Here's how the part is built. I have some questions about the finished solid (model axes, mm). A direction names the side the tool comes from. Round coordinates to 2 decimals unless told otherwise and drop trailing zeros. Write each loop counter-clockwise with the first axis right and the second up, starting at its lowest first coordinate (ties: lowest second). Pieces come first, ordered by that corner, then holes. Notation, with made-up numbers: (72, 59.5) - (108, 59.5) arc R4 ccw to (108, 65.5) - close; hole circle Ø2 at (43.5, 28.25). An arc over 180 degrees is marked (long way). One line per item, written item: value. Start each with the question number.
Item 1: For P1, Ø10, axis at x = 81, y = -48.5, coming from the +Z side; P2, Ø1.5, axis at y = -12.5, z = 15.5, coming from the +X side; P3, Ø1.5, axis at y = 14, z = 30, coming from the +X side; P4, Ø12, axis at y = -67.5, z = 10.5, coming from the +X side, each with a flat end and sliding along its axis, tell me the tip position at first contact or that it passes through.
Item 2: Imagine slicing it at B-B, the plane z = -13.5. Please give me the cut outline in (x, y).
Item 3: If I drill on line 1 (Z direction, x = -35, y = -20.5); line 2 (X direction, y = -64, z = 1); line 3 (Z direction, x = -42.5, y = -14.5), over which ranges is the centre line in solid material (lowest first)?
Item 4: Imagine slicing it at C-C, the plane x = 33.5. Please give me the cut outline in (y, z), then the cut area to 3 significant figures.
Item 5: Imagine slicing it at A-A, the plane y = 27. Please give me the cut outline in (x, z), then the cut area to 3 significant figures.
Item 6: Imagine slicing it at D-D, the plane x = -58. Please give me the cut outline in (y, z), then the cut area to 3 significant figures.
Item 7: Thinking about a two-plate mould opening in X: for faces 5 (the face through (59.417, -33.844, -12.525)), 6 (the face through (-30, 0, 28.945)), 7 (the face through (21.498, -69, 1)), which applies, released by +X, released by -X, zero draft, split by the parting line, or undercut?
Item 8: For faces 1 (the face through (-30, 16.289, 33)), 2 (the face through (53, -61.088, -4)), 3 (the face through (23.58, -33.81, -4.68)), 4 (the face through (0, -1, -16)), which set-ups out of +Z, -Z, +X, -X, +Y, -Y let a thin tool reach every point of the face, with its end or its side?
```python
from build123d import *

# Parameters (mm, degrees)
F1_DEPTH  = 76.2
F2_DEPTH  = 76.2
F3_W      = 72.8542578737
F3_H      = 12.1001238003
F4_DEPTH  = 152.401
F5_W      = 82.1163672954
F5_H      = 15.1120005071
F6_DEPTH  = 59.4443229417
F7_W      = 32.5772352517
F7_H      = 8.1773027778
F8_DEPTH  = 176.4699010899
F9_R      = 11.4001375148
F10_DEPTH = 59.4443229417
F11_R     = 12.1676085245
F12_DEPTH = 59.4443229417
F13_R     = 11.1566059008
F14_DEPTH = 59.4443229417
F15_R     = 11.1566059008
F16_DEPTH = 59.4443229417


with BuildPart() as f1:
    # F0 (on Front) → F1 (new body)
    with BuildSketch(Plane.XZ):
        Polygon((103.6146432161, -22.3206151277), (0, 37.122707814), (-72.8542578737, 37.122707814), (-72.8542578737, -22.3206151277), align=None)
    extrude(amount=F1_DEPTH)

    # F2 (add): a face of the model
    f2_faces = [f1.faces().sort_by_distance(p)[0] for p in [
        (-6.935088319, 0, 3.283766903),
    ]]
    extrude(f2_faces, amount=F2_DEPTH)

    # F3 (on face) → F4 (cut, through all)
    with BuildSketch(Plane.XZ.offset(76.2)):
        with Locations((-36.4271289369, -16.2705532275)):
            Rectangle(F3_W, F3_H)
    extrude(amount=-F4_DEPTH, mode=Mode.SUBTRACT)

    # F5 (on face) → F6 (cut, through all)
    with BuildSketch(Plane(origin=(0, 0, -22.3206151277), x_dir=(1, 0, 0), z_dir=(0, 0, -1))):
        with Locations((62.5564595684, 68.6439997464)):
            Rectangle(F5_W, F5_H)
    extrude(amount=-F6_DEPTH, mode=Mode.SUBTRACT)

    # F7 (on face) → F8 (cut, through all)
    with BuildSketch(Plane(origin=(-72.8542578737, 0, 0), x_dir=(0, -1, 0), z_dir=(-1, 0, 0))):
        with Locations((0, 33.0340564251)):
            Rectangle(F7_W, F7_H)
    extrude(amount=-F8_DEPTH, mode=Mode.SUBTRACT)

    # F9 (on face) → F10 (cut, through all)
    with BuildSketch(Plane(origin=(0, 0, -22.3206151277), x_dir=(1, 0, 0), z_dir=(0, 0, -1))):
        with Locations((34.9696464837, 33.3093106747)):
            Circle(F9_R)
    extrude(amount=-F10_DEPTH, mode=Mode.SUBTRACT)

    # F11 (on face) → F12 (cut, through all)
    with BuildSketch(Plane(origin=(0, 0, -22.3206151277), x_dir=(1, 0, 0), z_dir=(0, 0, -1))):
        with Locations((71.5732872486, 33.3093106747)):
            Circle(F11_R)
    extrude(amount=-F12_DEPTH, mode=Mode.SUBTRACT)

    # F13 (on face) → F14 (cut, through all)
    with BuildSketch(Plane(origin=(0, 0, -22.3206151277), x_dir=(1, 0, 0), z_dir=(0, 0, -1))):
        with Locations((35.3356823325, -35.1394936442)):
            Circle(F13_R)
    extrude(amount=-F14_DEPTH, mode=Mode.SUBTRACT)

    # F15 (on face) → F16 (cut, through all)
    with BuildSketch(Plane(origin=(0, 0, -22.3206151277), x_dir=(1, 0, 0), z_dir=(0, 0, -1))):
        with Locations((69.3770647049, -34.4074219465)):
            Circle(F15_R)
    extrude(amount=-F16_DEPTH, mode=Mode.SUBTRACT)


solid = f1.part
```
Values follow:
1. P1: stops at z = -6.48
1. P2: stops at x = 39
1. P3: passes through
1. P4: stops at x = 21.5
2. outline: (0, -76.2) - (21.5, -76.2) - (21.5, -61.09) - (88.24, -61.09) - (88.24, 76.2) - (0, 76.2) - close; hole circle Ø22.8 at (34.97, -33.31); hole circle Ø22.31 at (35.34, 35.14); hole circle Ø22.31 at (69.38, 34.41); hole circle Ø24.34 at (71.57, -33.31)
3. line 1: z = -10.22 to 37.12
3. line 2: x = -72.85 to 21.5
3. line 3: z = -10.22 to 28.95
4. outline: (-61.09, -22.32) - (-44.61, -22.32) - (-44.61, 17.9) - (-61.09, 17.9) - close; (-22, -22.32) - (24.13, -22.32) - (24.13, 17.9) - (-22, 17.9) - close; (46.14, -22.32) - (76.2, -22.32) - (76.2, 17.9) - (46.14, 17.9) - close
4. area: 3,730 mm^2
5. outline: (-72.85, -10.22) - (0, -10.22) - (0, -22.32) - (27.71, -22.32) - (27.71, 21.23) - (0, 37.12) - (-72.85, 37.12) - close; (42.97, -22.32) - (61.03, -22.32) - (61.03, 2.11) - (42.97, 12.47) - close; (77.72, -22.32) - (103.61, -22.32) - (77.72, -7.46) - close
5. area: 5,600 mm^2
6. outline: (-76.2, -10.22) - (76.2, -10.22) - (76.2, 37.12) - (16.29, 37.12) - (16.29, 28.95) - (-16.29, 28.95) - (-16.29, 37.12) - (-76.2, 37.12) - close
6. area: 6,950 mm^2
7. face 5: undercut
7. face 6: zero draft
7. face 7: released by +X
8. face 1: +Z, +X, -X
8. face 2: +Z, -Z, +X, -Y
8. face 3: +Z, -Z
8. face 4: -Z, -X, +Y, -Y
